Design review of the part built by this model. Coordinates are the model's own, in mm. Round coordinates to 2 decimals unless told otherwise and drop trailing zeros. Order: outer loops, then holes, each group sorted by start corner. A loop starts at its lowest first (then second) coordinate and runs counter-clockwise, first axis right, second up. Notation, with made-up numbers: (-26.5, -16) - (5.5, -16) arc R17 ccw to (5.5, 8) - close; hole circle Ø8 at (60, -8). An arc over 180 degrees is marked (long way). Answer as a JSON object with one key per item and string values. Group by question number.
from build123d import *

# Parameters (mm, degrees)
SKETCH1_W           = 25.4
SKETCH1_H           = 25.4
BOSS_EXTRUDE1_DEPTH = 63.5
SKETCH2_R           = 6.35
CUT_EXTRUDE1_DEPTH  = 26.4


with BuildPart() as part:
    # Sketch1 → Boss-Extrude1 (new body)
    with BuildSketch(Plane.XY):
        with Locations((-17.064491321, 20.342163666)):
            Rectangle(SKETCH1_W, SKETCH1_H)
    extrude(amount=BOSS_EXTRUDE1_DEPTH)

    # Sketch2 → Cut-Extrude1 (cut, through all)
    with BuildSketch(Plane.ZY.offset(29.764491321)):
        with Locations((50.8, 20.342163666)):
            Circle(SKETCH2_R)
    extrude(amount=-CUT_EXTRUDE1_DEPTH, mode=Mode.SUBTRACT)


solid = part.part
1. To check wall thickness, follow line 1 (Y direction, x = -14.25, z = 50.8); line 2 (Z direction, x = -24.5, y = 21.25); line 3 (Z direction, x = -14.5, y = 25.5). State the ranges of each line that lie inside material, in increasing order. Write a range as from..to.
2. Clearance check with a flat-ended pin moving along its axis: P1, Ø1, axis at x = -8, y = 26.5, coming from the -Z side. State where the tip first meets the part, or that it passes through.
3. Mouldability with a two-part tool opening along Z and no side actions: class faces 1 (the flat face through (-17, 21, 63.5)), 2 (the cylindrical face through (-17.24, 14.71, 53.73)), 3 (the flat face through (-17, 21, 0)), 4 (the flat face through (-17, 7.642, 31)) as pulls with the +Z half, pulls with the -Z half, needs draft (parallel to the pull), parting line crosses it, or undercut.
4. Take a section at C-C, the plane x = -24.25. Give the boundary of the cut face in (y, z).
5. Take a section at B-B, the plane y = 16.5. Give the boundary of the cut face in (x, z).
6. Take a section at A-A, the plane z = 50.8. Give the boundary of the cut face in (x, y), then the cut area to 3 significant figures.
Response values:
{
 "1": {"line 1": "7.64..13.99, 26.69..33.04", "line 2": "0..44.52, 57.08..63.5", "line 3": "0..47.1, 54.5..63.5"},
 "2": {"P1": "z = 0"},
 "3": {"face 1": "pulls with the +Z half", "face 2": "undercut", "face 3": "pulls with the -Z half", "face 4": "needs draft"},
 "4": {"outline": "(7.64, 0) - (33.04, 0) - (33.04, 63.5) - (7.64, 63.5) - close; hole circle Ø12.7 at (20.34, 50.8)"},
 "5": {"outline": "(-29.76, 0) - (-4.36, 0) - (-4.36, 45.74) - (-29.76, 45.74) - close; (-29.76, 55.86) - (-4.36, 55.86) - (-4.36, 63.5) - (-29.76, 63.5) - close"},
 "6": {"outline": "(-29.76, 7.64) - (-4.36, 7.64) - (-4.36, 13.99) - (-29.76, 13.99) - close; (-29.76, 26.69) - (-4.36, 26.69) - (-4.36, 33.04) - (-29.76, 33.04) - close", "area": "323 mm2"}
}
